Can you work these out from the drawing? Everything is in mm from the part's minimum corner. A direction names the side the tool comes from. Give positions to 0.01 mm unless a question says otherwise; leave off trailing zeros. Order: outer loops, then holes, each group sorted by start corner. A loop starts at its lowest first (then second) coordinate and runs counter-clockwise, first axis right, second up. Notation, with made-up numbers: (-36, -11.5) -> (-12, -11.5) arc R11 ccw to (-12, -0.5) -> close; hole circle Ø3 at (2.25, 60.25). An arc over 180 degrees is marked (long way). Answer as CSV lines item,"result". Start each with the question number.
(1) I want a section at D-D (x = 15.25). Please give me the cut outline in (y, z), plus the area to 3 significant figures.
(2) I want a section at B-B (y = 12.5). Please give me the cut outline in (x, z).
(3) Will these pins go through, and if not, where does the flat tip stop? pin 1 Ø10 at (x, y) = (5.5, 18) entering from -Z; pin 2 Ø1 at (x, z) = (7, 7.5) entering from -Y; pin 3 Ø3 at (x, z) = (10, 3) entering from -Y; pin 4 Ø10 at (x, y) = (6.5, 7) entering from +Z.
(4) I need wall thicknesses on L1, parallel to Z at x = 9, y = 6.5; L2, parallel to Y at x = 10.75, z = 6 (1 decimal); L3, parallel to Y at x = 14.25, z = 5.75 (1 decimal). Which ranges of each line are inside material? Lowest first, please.
(5) I want a section at C-C (z = 2.75). Please give me the cut outline in (x, y).
(6) I want a section at A-A (x = 3). Please give me the cut outline in (y, z), plus the area to 3 significant figures.
(7) On a 3-axis mill with a long thin cutter (end or side, diameter ignored), from which of +Z, -Z, +X, -X, +Y, -Y can I reach the whole of each face in a straight line? I mean the marked faces 1 and 2. Say none if no direction works.
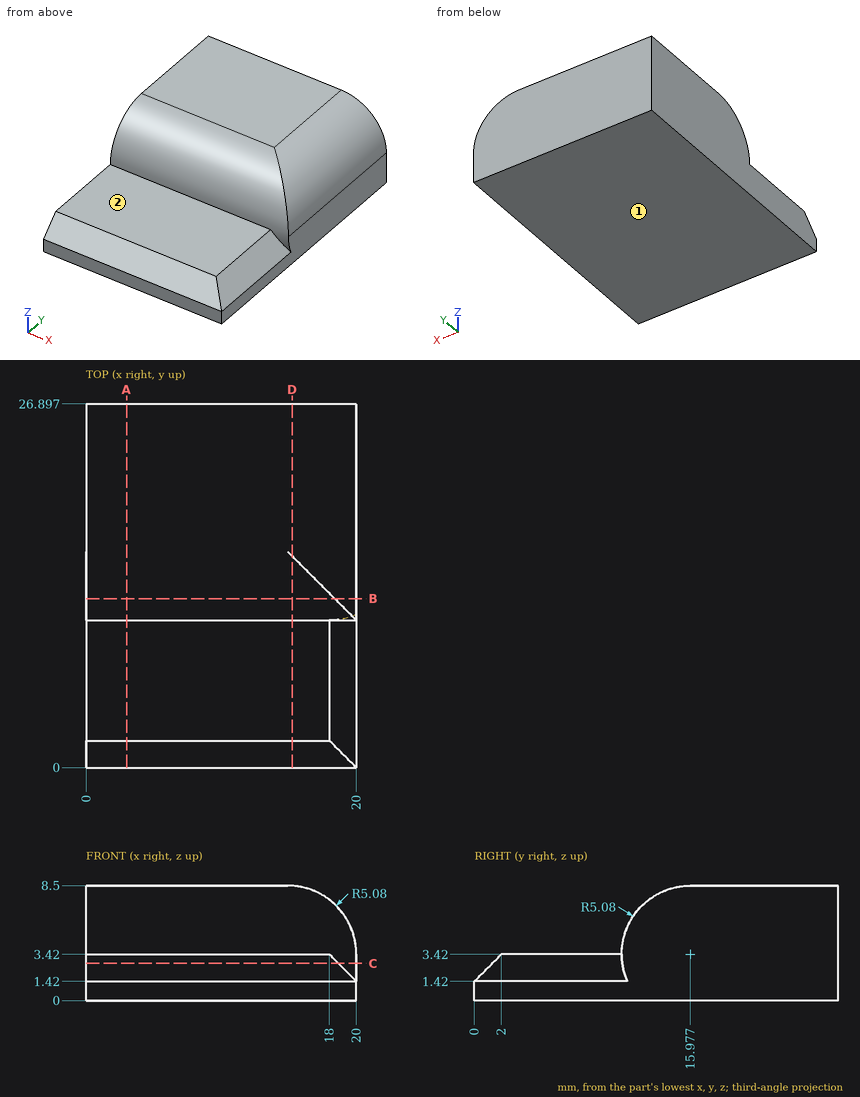
Final values:
1,outline,"(0, 0) -> (26.9, 0) -> (26.9, 8.49) -> (15.65, 8.49) arc R5.08 ccw to (10.9, 3.42) -> (2, 3.42) -> (0, 1.42) -> close"
1,area,"166 mm²"
2,outline,"(0, 0) -> (20, 0) -> (20, 3.42) arc R5.08 ccw to (18.4, 7.12) -> (0, 7.12) -> close"
3,pin 1,"z = 0"
3,pin 2,"y = 12.37"
3,pin 3,"y = 0.08"
3,pin 4,"z = 6.58"
4,L1,"0 to 3.42"
4,L2,"11.6 to 26.9"
4,L3,"11.5 to 26.9"
5,outline,"(0, 1.33) -> (18.67, 1.33) -> (18.67, 10.94) -> (20, 10.94) -> (20, 26.9) -> (0, 26.9) -> close"
6,outline,"(0, 0) -> (26.9, 0) -> (26.9, 8.5) -> (15.98, 8.5) arc R5.08 ccw to (10.9, 3.42) -> (2, 3.42) -> (0, 1.42) -> close"
6,area,"166 mm²"
7,face 1,"-Z, +X, -X, +Y, -Y"
7,face 2,"+Z, +X, -X, -Y"
